Geometry: final body of the model. Coordinates: model frame, mm. A direction names the side the tool comes from. Give positions to 0.01 mm unless a question says otherwise; leave off trailing zeros. Write each loop counter-clockwise with the first axis right and the second up, starting at its lowest first coordinate (ties: lowest second). Pieces come first, ordered by that corner, then holes. Notation, with made-up numbers: M 41,44.25 L 58,44.25 A15 ccw 58,71.25 Z; hole C 5,11.5 d7. An arc over 180 degrees is marked long. Use one line per item in the form item = value. Start each with the question number.
Item 1: Material intervals for line 1 along X through (y, z) = (3, 2.75); line 2 along Y through (x, z) = (12.75, 6.75); line 3 along Y through (x, z) = (12.5, 4.75), sorted ascending. Write a range as from..to.
Item 2: Section query B-B on x = -4.75. Return loops of the section in (y, z).
Item 3: Section query D-D on x = -1. Return loops of the section in (y, z).
Item 4: Section query C-C on y = -3.75. Return loops of the section in (x, z), then the cut area to 3 significant figures.
Item 5: Access query for faces 1 (the flat face through (-9, 13, 4)), 2 (the flat face through (8, 0, 2.8)). Directions: +Z, -Z, +X, -X, +Y, -Y. A direction counts if a zero-diameter tool reaches every point of the face in a straight line with its end or side. Return the directions, or none.
Item 6: Pull-direction query (Y, two-part tool) for faces 3 (the flat face through (0, -15, 3)), 4 (the flat face through (-4, -14.5, 6)), 5 (the flat face through (9, -13, 4)), 6 (the flat face through (9, 13, 4)); classes: released by +Y, released by -Y, zero draft, split by the parting line, or undercut.
Item 7: Section query A-A on z = 7. Return loops of the section in (x, y), then the cut area to 3 significant figures.
Item 8: Contact query for flat-ended pins moving along their axis: P1, Ø1.5, axis at x = -11.5, y = 11, coming from the +Z side; P2, Ø4, axis at x = 0, y = -4.5, coming from the +Z side. Output: stop coordinate, or through.
from build123d import *

# Parameters (mm, degrees)
SKETCH_W            = 30
SKETCH_H            = 30
PAD_DEPTH           = 3.5
POCKET_DEPTH        = 30.001
LINEARPATTERN_COUNT = 2
LINEARPATTERN_PITCH = 15
SKETCH002_W         = 30
SKETCH002_H         = 30
SKETCH002_W_2       = 28
SKETCH002_H_2       = 28
PAD001_DEPTH        = 5
PAD002_DEPTH        = 2
POLARPATTERN_COUNT  = 4
SKETCH004_W         = 8
SKETCH004_H         = 5
POCKET001_DEPTH     = 1


with BuildPart() as part:
    # Sketch → Pad (new body)
    with BuildSketch(Plane.XY):
        Rectangle(SKETCH_W, SKETCH_H)
    extrude(amount=PAD_DEPTH)

    # Sketch001 → Pocket (cut, through all)
    with BuildSketch(Plane(origin=(0, 15, 0), x_dir=(-1, 0, 0), z_dir=(0, 1, 0))):
        with BuildLine():
            Line((-9, 0.722949), (-9, 0))
            Line((-9, 0), (-6, 0))
            Line((-6, 0), (-6, 0.722949))
            ThreePointArc((-6, 0.722949), (-5.37226, 1.668412), (-5.285841, 2.8))
            Line((-9.714159, 2.8), (-5.285841, 2.8))
            ThreePointArc((-9.714159, 2.8), (-9.62774, 1.668412), (-9, 0.722949))
        make_face()
    pocket = extrude(amount=-POCKET_DEPTH, mode=Mode.SUBTRACT)

    # LinearPattern: Pocket ×2
    with Locations(*[(-i * LINEARPATTERN_PITCH, 0, 0) for i in range(1, LINEARPATTERN_COUNT)]):
        add(pocket, mode=Mode.SUBTRACT)

    # Sketch002 → Pad001 (new body)
    with BuildSketch(Plane.XY.offset(3.5)):
        Rectangle(SKETCH002_W, SKETCH002_H)
        Rectangle(SKETCH002_W_2, SKETCH002_H_2, mode=Mode.SUBTRACT)
    extrude(amount=PAD001_DEPTH)

    # Sketch003 → Pad002 (new body)
    with BuildSketch(Plane.XY.offset(3.5)):
        with BuildLine():
            Line((-14, 14), (-14, 9))
            Line((-14, 9), (-11.5, 9))
            ThreePointArc((-11.5, 9), (-9.732233, 9.732233), (-9, 11.5))
            Line((-9, 14), (-9, 11.5))
            Line((-14, 14), (-9, 14))
        make_face()
    pad002 = extrude(amount=PAD002_DEPTH)

    # PolarPattern: Pad002 ×4 about axis
    polarpattern_axis = Axis((0, 0, 3.5), (0, 0, 1))
    for i in range(1, POLARPATTERN_COUNT):
        add(pad002.rotate(polarpattern_axis, i * 360 / POLARPATTERN_COUNT))

    # Sketch004 → Pocket001 (cut)
    with BuildSketch(Plane.XZ.offset(15)):
        with Locations((0, 6)):
            Rectangle(SKETCH004_W, SKETCH004_H)
    extrude(amount=-POCKET001_DEPTH, mode=Mode.SUBTRACT)


solid = part.part
Answer sheet:
q1.line_1 = -15..-9.72, -5.28..5.28, 9.72..15
q1.line_2 = -15..-14, 14..15
q1.line_3 = -15..-9, 9..15
q2.outline = M -15,0 L 15,0 L 15,8.5 L 14,8.5 L 14,3.5 L -14,3.5 L -14,8.5 L -15,8.5 Z
q3.outline = M -15,0 L 15,0 L 15,8.5 L 14,8.5 L 14,3.5 L -15,3.5 Z
q4.outline = M -15,0 L -9,0 L -9,0.72 A2.25 cw -9.71,2.8 L -5.29,2.8 A2.25 cw -6,0.72 L -6,0 L 6,0 L 6,0.72 A2.25 cw 5.29,2.8 L 9.71,2.8 A2.25 cw 9,0.72 L 9,0 L 15,0 L 15,8.5 L 14,8.5 L 14,3.5 L -14,3.5 L -14,8.5 L -15,8.5 Z
q4.area = 93.5 mm2
q5.face_1 = +Z
q5.face_2 = +Y, -Y
q6.face_3 = released by -Y
q6.face_4 = zero draft
q6.face_5 = undercut
q6.face_6 = undercut
q7.outline = M -15,-15 L -4,-15 L -4,-14 L -14,-14 L -14,14 L 14,14 L 14,-14 L 4,-14 L 4,-15 L 15,-15 L 15,15 L -15,15 Z
q7.area = 108 mm2
q8.P1 = 5.5
q8.P2 = 3.5
